Verification items for this drawing (mm, ordinates from the low corner). A direction names the side the tool comes from. Coordinates: 2 decimals unless noted, no trailing zeros. Order: outer loops, then holes, each group sorted by start corner. A loop starts at its lowest first (then second) coordinate and runs counter-clockwise, first axis right, second up. Notation, with made-up numbers: M 54.25,77.5 L 71.25,77.5 A22 cw 71.25,100.5 Z; hole C -2,-32.75 d9. An arc over 180 degrees is marked long. One line per item, written item: value. Start each with the question number.
1) Sectioned sample at D-D, the plane y = 64. Enter the section's corners in (x, z) (1 decimal).
2) Thickness scan on L1, parallel to X at y = 70, z = 33; L2, parallel to Y at x = 28, z = 60; L3, parallel to X at y = 69.5, z = 33.5. Record the ranges inside material, lowest first. Write a range as from..to.
3) Sectioned sample at C-C, the plane y = 28. Enter the section's corners in (x, z) (1 decimal).
4) Go/stop test with flat-tipped pins: P1, Ø1.5, axis at x = 33, y = 87, coming from the -Z side; P2, Ø8, axis at y = 133, z = 39, coming from the +X side; P3, Ø3, axis at x = 53.5, z = 47, coming from the -Y side (1 decimal). Record where each tip stops, or that it passes through.
5) Sectioned sample at A-A, the plane y = 134. Enter the section's corners in (x, z) (1 decimal), then the cut area to 3 significant figures.
6) Access from +Z, -Z, +X, -X, +Y, -Y to the whole of each face (thin tool, end or side, straight path). Record for the marked faces 1 and 2.
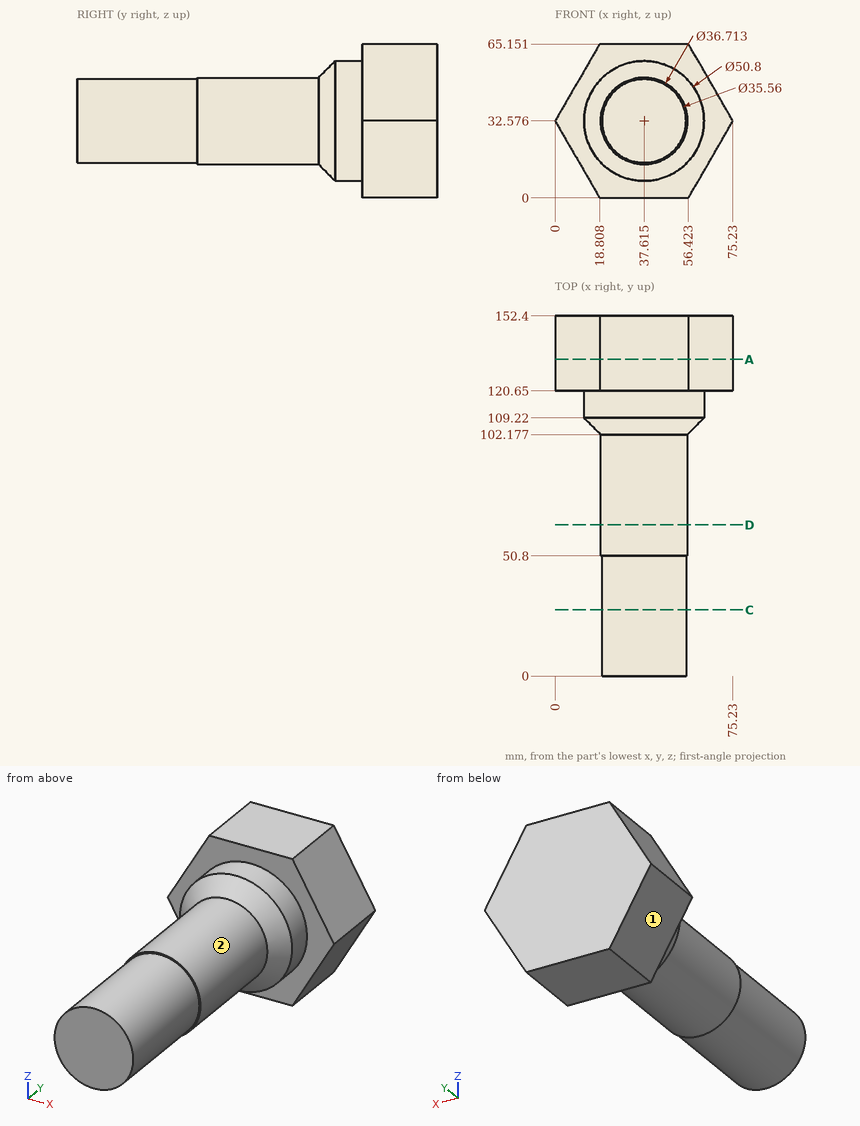
Final values:
1. outline: C 37.6,32.6 d36.7
2. L1: x = 19.26..55.97
2. L2: y = 120.65..152.4
2. L3: x = 19.28..55.95
3. outline: C 37.6,32.6 d35.6
4. P1: stops at z = 14.63
4. P2: stops at x = 73.83
4. P3: stops at y = 103.8
5. outline: M 0,32.6 L 18.8,0 L 56.4,0 L 75.2,32.6 L 56.4,65.2 L 18.8,65.2 Z
5. area: 3,680 mm^2
6. face 1: -Z, -X, +Y, -Y
6. face 2: -Y
